from build123d import *

# Parameters (mm, degrees)
SKETCH1_R           = 3.3
BOSS_EXTRUDE3_DEPTH = 2.54
FILLET1_R           = 2.54
FILLET2_R           = 2.54


with BuildPart() as part:
    # Sketch1 → Boss-Extrude3 (new body)
    with BuildSketch(Plane.XY):
        with BuildLine():
            Line((32.190295112, -35.281999932), (-9.173256028, -10.079873667))
            Line((-9.173256028, -10.079873667), (6.764957958, 12.279616129))
            Line((6.764957958, 12.279616129), (43.439198939, -19.997724209))
            ThreePointArc((43.439198939, -19.997724209), (44.817595988, -32.793810869), (32.190295112, -35.281999932))
        make_face()
        with Locations((37.146277839, -27.14788288)):
            Circle(SKETCH1_R, mode=Mode.SUBTRACT)
    extrude(amount=BOSS_EXTRUDE3_DEPTH)

    # Fillet1
    fillet1_edges = [part.edges().sort_by_distance(p)[0] for p in [
        (-9.173256028, -10.079873667, 1.27),
    ]]
    fillet(fillet1_edges, radius=FILLET1_R)

    # Fillet2
    fillet2_edges = [part.edges().sort_by_distance(p)[0] for p in [
        (6.764957958, 12.279616129, 1.27),
    ]]
    fillet(fillet2_edges, radius=FILLET2_R)


solid = part.part
The model under review builds one solid part; all positions refer to its coordinate system, in mm. Round coordinates to 2 decimals unless told otherwise and drop trailing zeros. Write each loop counter-clockwise with the first axis right and the second up, starting at its lowest first coordinate (ties: lowest second). Pieces come first, ordered by that corner, then holes. Notation, with made-up numbers: (42, -30) - (47, -30) arc R30 ccw to (47, 6) - close; hole circle Ø1 at (-20, 84.25). An arc over 180 degrees is marked (long way). One line per item, written item: value. Start each with the question number.
1. Consider section B-B on z = 0.6. Write out the cut boundary in (x, y) (3 decimals).
2. Clearance check with flat-ended pins moving along their axes: P1, Ø1, axis at x = 14, z = 0.5, coming from the +Y side; P2, Ø1, axis at x = 13, z = 2, coming from the -Y side; P3, Ø1, axis at x = 12, z = 2, coming from the +Y side. State where each tip first meets the part, or that it passes through.
3. Consider section A-A on y = -28.5. Write out the cut boundary in (x, z), and give its area (3 significant figures).
4. Consider section D-D on y = -5. Write out the cut boundary in (x, z).
5. The part is to be moulded in two halves that separate along X. For faces 1 (the face through (6.879, 11.033, 1.288)), 2 (the face through (-8.003, -9.87, 1.288)), 3 (the face through (40.294, -26.157, 1.252)), say which applies: released by +X, released by -X, zero draft, split by the parting line, or undercut.
6. Consider section C-C on x = 39.5. Write out the cut boundary in (y, z).
7. To check wall thickness, follow L1, parallel to Y at x = 38.5, z = 1.5; L2, parallel to Y at x = 40, z = 0.55; L3, parallel to Y at x = 2.5, z = 2.25. State the ranges of each line that lie inside material, in increasing order. Write a range as from..to.
Checks:
1. outline: (-7.589, -7.857) arc R2.54 ccw to (-6.842, -11.5) - (32.19, -35.282) arc R9.525 ccw to (43.439, -19.998) - (8.878, 10.42) arc R2.54 ccw to (5.131, 9.988) - close; hole circle Ø6.6 at (37.146, -27.148)
2. P1: stops at y = 6.35
2. P2: stops at y = -23.89
2. P3: stops at y = 8.11
3. outline: (21.06, 0) - (34.14, 0) - (34.14, 2.54) - (21.06, 2.54) - close; (40.16, 0) - (46.57, 0) - (46.57, 2.54) - (40.16, 2.54) - close
3. area: 49.5 mm^2
4. outline: (-5.55, 0) - (26.4, 0) - (26.4, 2.54) - (-5.55, 2.54) - close
5. face 1: split by the parting line
5. face 2: released by -X
5. face 3: undercut
6. outline: (-36.38, 0) - (-29.46, 0) - (-29.46, 2.54) - (-36.38, 2.54) - close; (-24.83, 0) - (-16.53, 0) - (-16.53, 2.54) - (-24.83, 2.54) - close
7. L1: y = -36.58..-30.16, -24.14..-15.65
7. L2: y = -36.24..-28.81, -25.49..-16.97
7. L3: y = -17.19..6.3
